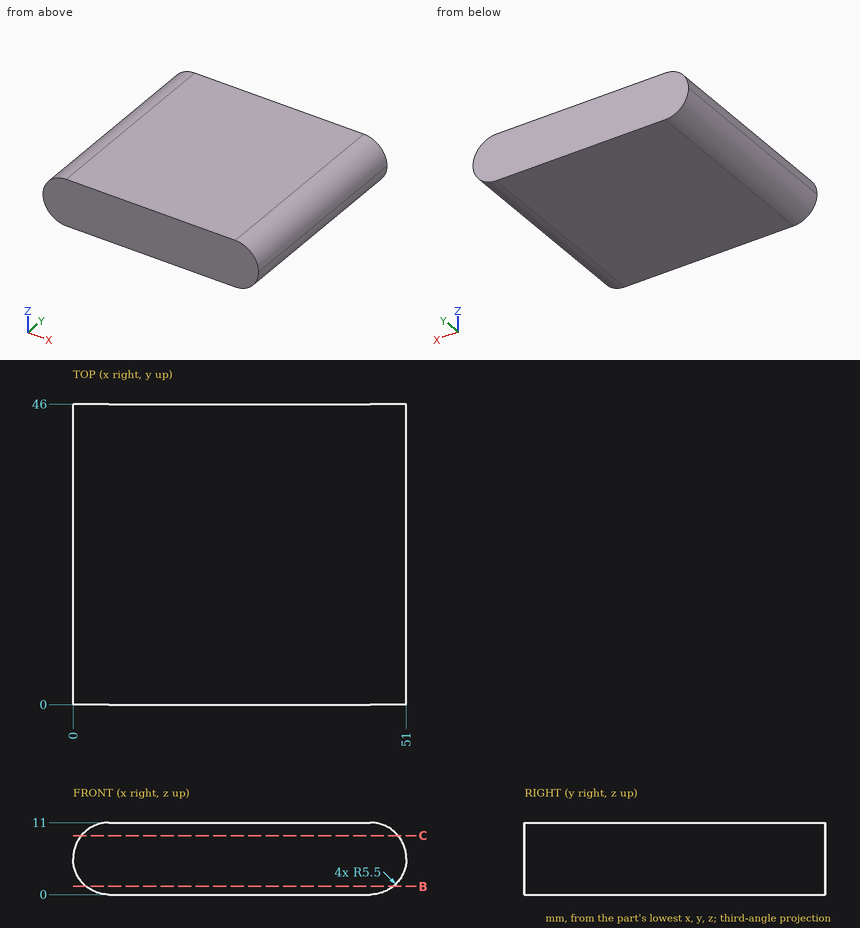
Design review of the part shown in the three views and the two pictorial views. Dimensions are in mm from the part's minimum x, y and z. Give positions to 0.01 mm unless a question says otherwise; leave off trailing zeros. Loops run counter-clockwise (first coordinate to the right, second up) from the corner with the lowest first, then second, coordinate; pieces in that order, holes last. Notation, with made-up numbers: (12.5, -7) - (48.5, -7) arc R35 ccw to (48.5, 25) - close; hole circle Ø7 at (1, -0.75). An arc over 180 degrees is marked (long way). Write item = value, one per line.
1) Clearance check with flat-ended pins moving along their axes: pin 1 Ø1.5 at (y, z) = (28.5, 2) entering from -X; pin 2 Ø3 at (x, y) = (36, 24.5) entering from -Z; pin 3 Ø1 at (y, z) = (36, 3.5) entering from +X. State where each tip first meets the part, or that it passes through.
Result sheet:
pin_1 = 0.74
pin_2 = 0
pin_3 = 50.79
2) Take a section at C-C on z = 9. State the section outline as (x, y) points, and give its area (3 significant figures).
Result sheet:
outline = (1.26, 0) - (49.74, 0) - (49.74, 46) - (1.26, 46) - close
area = 2,230 mm2
3) To check wall thickness, follow line 1 (X direction, y = 32, z = 4.25); line 2 (Z direction, x = 5, y = 21); line 3 (X direction, y = 8.5, z = 1.5) (1 decimal). State the ranges of each line that lie inside material, in increasing order.
Result sheet:
line_1 = 0.14 to 50.86
line_2 = 0.02 to 10.98
line_3 = 1.7 to 49.3
4) Take a section at B-B on z = 1.25. State the section outline as (x, y) points, and give its area (3 significant figures).
Result sheet:
outline = (2.01, 0) - (48.99, 0) - (48.99, 46) - (2.01, 46) - close
area = 2,160 mm2
